from build123d import *

# Parameters (mm, degrees)
EXTRUDE_1_DEPTH     = 11
EXTRUDE_1_2_DEPTH   = 11
EXTRUDE_2_DEPTH     = 2
SKETCH_5_W          = 30
SKETCH_5_H          = 38
SKETCH_5_W_2        = 18
SKETCH_5_H_2        = 26
EXTRUDE_3_DEPTH     = 2
SKETCH_6_R          = 1.5
CUT_EXTRUDE_1_DEPTH = 27.245152284


with BuildPart() as part:
    # Sketch 1 → Extrude 1 (new, symmetric)
    with BuildSketch(Plane(origin=(0, 0, 0), x_dir=(1, 0, 0), z_dir=(0, 1, 0))):
        with BuildLine():
            Line((-9, 30), (-9, 24.924887161))
            ThreePointArc((-9, 24.924887161), (0, 26.5), (9, 24.924887161))
            Line((9, 24.924887161), (9, 30))
            Line((9, 30), (-9, 30))
        make_face()
    extrude(amount=EXTRUDE_1_DEPTH, both=True)



with BuildPart() as body_2:
    # Sketch 1 → Extrude 1 2 (new, symmetric)
    with BuildSketch(Plane(origin=(0, 0, 0), x_dir=(1, 0, 0), z_dir=(0, 1, 0))):
        with BuildLine():
            Line((-9, 20.0748599), (-9, 17.860571099))
            ThreePointArc((-9, 17.860571099), (0, 20), (9, 17.860571099))
            Line((9, 17.860571099), (9, 20.0748599))
            ThreePointArc((9, 20.0748599), (0, 22), (-9, 20.0748599))
        make_face()
    extrude(amount=EXTRUDE_1_2_DEPTH, both=True)


with BuildPart() as part_1:
    add(part.part)

    add(body_2.part)  # Extrude 2 merges body 2
    # Sketch 2 → Extrude 2 (add)
    with BuildSketch(Plane(origin=(0, 11, 0), x_dir=(1, 0, 0), z_dir=(0, 1, 0))):
        with BuildLine():
            Line((-9, 30), (-9, 17.860571099))
            ThreePointArc((-9, 17.860571099), (0, 20), (9, 17.860571099))
            Line((9, 17.860571099), (9, 30))
            Line((9, 30), (-9, 30))
        make_face()
    extrude_2 = extrude(amount=EXTRUDE_2_DEPTH)

    # Mirror 1: Extrude 2 across plane
    add(extrude_2.mirror(Plane.ZX))

    # Sketch 5 → Extrude 3 (add)
    with BuildSketch(Plane(origin=(0, 0, -30), x_dir=(-1, 0, 0), z_dir=(0, 0, -1))):
        Rectangle(SKETCH_5_W, SKETCH_5_H)
        Rectangle(SKETCH_5_W_2, SKETCH_5_H_2, mode=Mode.SUBTRACT)
    extrude(amount=-EXTRUDE_3_DEPTH)

    # Sketch 6 → Cut-Extrude 1 (cut, through all)
    with BuildSketch(Plane.XY.offset(-28)):
        with Locations((12, 16)):
            Circle(SKETCH_6_R)
        with Locations(Location((-12, 16, 0), (0, 0, 180))):
            Circle(SKETCH_6_R)
        with Locations(Location((12, -16, 0), (0, 0, 180))):
            Circle(SKETCH_6_R)
        with Locations((-12, -16)):
            Circle(SKETCH_6_R)
    extrude(amount=-CUT_EXTRUDE_1_DEPTH, mode=Mode.SUBTRACT)


solid = part_1.part
Model file for the job. Use its own axes, mm. A direction names the side the tool comes from. Give positions to 0.01 mm unless a question says otherwise; leave off trailing zeros. Order: outer loops, then holes, each group sorted by start corner. A loop starts at its lowest first (then second) coordinate and runs counter-clockwise, first axis right, second up. Notation, with made-up numbers: (-4, 57) - (23, 57) arc R37 ccw to (23, 94) - close; hole circle Ø11 at (67, 1). An arc over 180 degrees is marked (long way). Write item = value, one per line. Start each with the question number.
1. Cut at B-B, the plane z = -25.75. List the corners of the cut face in (x, y), and give its area (3 significant figures).
2. Which spindle directions (+Z, -Z, +X, -X, +Y, -Y) get a long thin tool onto all of the face, cutting with end or side? Do faces 4 (the flat face through (0, -13, -24)), 5 (the flat face through (0, 11, -23)), 6 (the flat face through (-9, 0.2, -25.3)). Say none if no direction does.
3. Probe line 1 along Y through (x, z) = (-1.5, -25); line 2 along Y through (x, z) = (-12, -28.9); line 3 along Z through (x, y) = (-9.25, -16.5). List the from-to ranges inside material, lowest first.
4. Cut at A-A, the plane x = -12. List the corners of the cut face in (y, z).
5. Cut at C-C, the plane y = -5. List the corners of the cut face in (x, z).
6. Two-plate mould, pull along X, no slides. Class faces 1 (the cylindrical face through (-10.5, 15.93, -28.99)), 2 (the flat face through (-15, 0, -29)), 3 (the flat face through (0, 13, -24)): pulls with the +X half, pulls with the -X half, needs draft (parallel to the pull), parting line crosses it, or undercut.
7. Cut at D-D, the plane y = -16. List the corners of the cut face in (x, z), and give its area (3 significant figures).
8. Drop flat-ended pins along their axis: P1, Ø6, axis at y = -10.5, z = -23.5, coming from the +X side; P2, Ø4, axis at y = -14, z = -27, coming from the +X side; P3, Ø3, axis at x = 4.5, z = -22, coming from the -Y side; P4, Ø3, axis at x = -9.5, z = -25.5, coming from the +Y side. Give the stop position or say it passes through.
Taken from the geometry:
q1.outline = (-9, -13) - (9, -13) - (9, 13) - (-9, 13) - close; hole (-6.26, -11) - (6.26, -11) - (6.26, 11) - (-6.26, 11) - close
q1.area = 193 mm²
q2.face_4 = +Z, +X, -X, -Y
q2.face_5 = none
q2.face_6 = +Z, -X, +Y, -Y
q3.line_1 = -13 to -11, 11 to 13
q3.line_2 = -19 to -17.5, -14.5 to 14.5, 17.5 to 19
q3.line_3 = -30 to -28
q4.outline = (-19, -30) - (-17.5, -30) - (-17.5, -28) - (-19, -28) - close; (-14.5, -30) - (14.5, -30) - (14.5, -28) - (-14.5, -28) - close; (17.5, -30) - (19, -30) - (19, -28) - (17.5, -28) - close
q5.outline = (-15, -30) - (15, -30) - (15, -28) - (9, -28) - (9, -24.92) arc R26.5 cw to (-9, -24.92) - (-9, -28) - (-15, -28) - close; (-9, -20.07) arc R22 ccw to (9, -20.07) - (9, -17.86) arc R20 cw to (-9, -17.86) - close
q6.face_1 = undercut
q6.face_2 = pulls with the -X half
q6.face_3 = needs draft
q7.outline = (-15, -30) - (-13.5, -30) - (-13.5, -28) - (-15, -28) - close; (-10.5, -30) - (10.5, -30) - (10.5, -28) - (-10.5, -28) - close; (13.5, -30) - (15, -30) - (15, -28) - (13.5, -28) - close
q7.area = 48.0 mm²
q8.P1 = 9
q8.P2 = 15
q8.P3 = -13
q8.P4 = 13
